Geometry: see drawing. Coordinates: mm, zero at the bounding-box minimum. A direction names the side the tool comes from. Give positions to 0.01 mm unless a question says otherwise; leave off trailing zeros. Write each loop counter-clockwise with the first axis right and the second up, starting at its lowest first coordinate (ties: lowest second). Pieces come first, ordered by that corner, then holes. Notation, with made-up numbers: (61.25, 33) -> (104.25, 33) arc R17 cw to (104.25, 54) -> close; hole circle Ø11 at (-9.75, -10.5). An arc over 180 degrees is marked (long way). Answer as a JSON object with one key per item and string values. Group by question number.
Item 1: Section query A-A on x = 4.5. Return the cut outline in (y, z).
Item 2: Section query C-C on y = 80. Return the cut outline in (x, z), plus the area to 3 significant figures.
Item 3: Access query for the marked faces 1 and 2. Directions: +Z, -Z, +X, -X, +Y, -Y. A direction counts if a zero-diameter tool reaches every point of the face in a straight line with its end or side. Return the directions, or none.
Item 4: First-contact query: pin 1 Ø10 at (x, y) = (35, 77.5) entering from +Z; pin 2 Ø5 at (x, y) = (39, 31.5) entering from +Z; pin 3 Ø20.5 at (x, z) = (37.5, 94) entering from -Y. Flat tips, straight axial feed; report the tip coordinate or a pass-through.
Item 5: Ray query, probe 1 along Y at (x, z) = (42, 86); probe 2 along Z at (x, y) = (31.5, 36); probe 3 along Y at (x, z) = (3, 72.5). Return the intervals inside material, ascending. Write a range as from..to.
Item 6: Section query B-B on z = 93.5. Return the cut outline in (x, y).
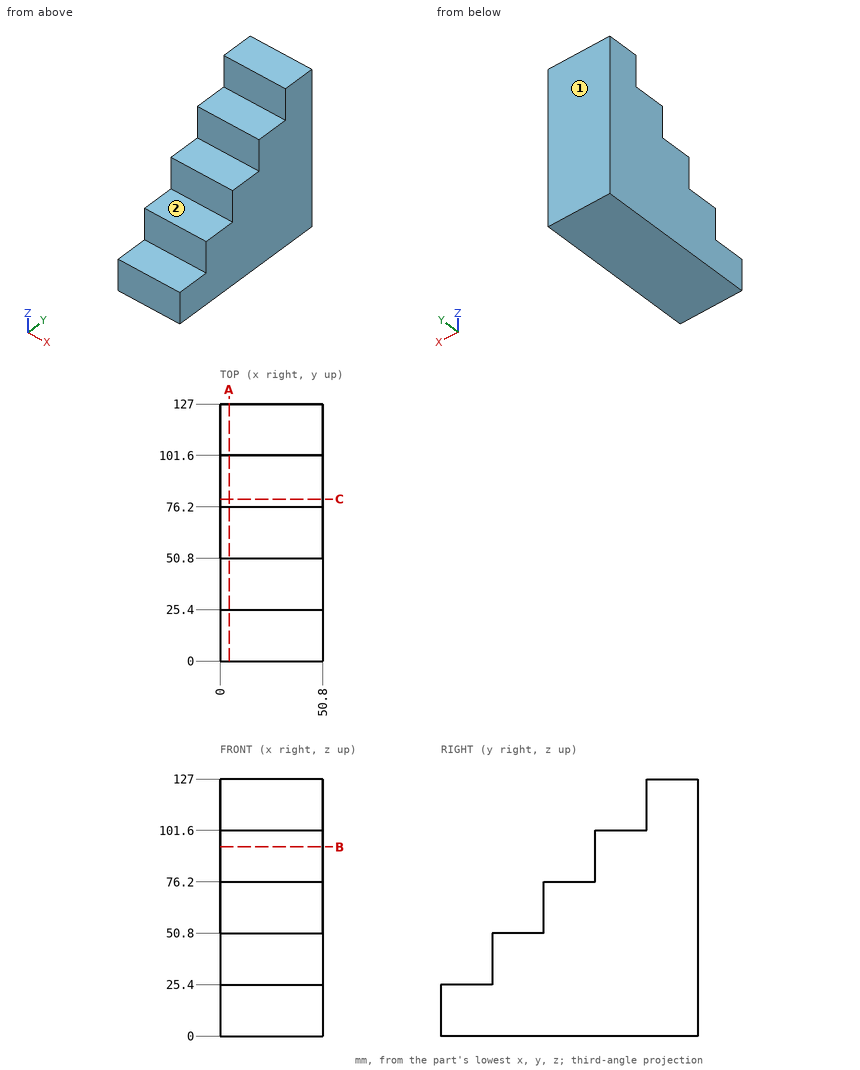
Worked answers:
{
 "1": {"outline": "(0, 0) -> (127, 0) -> (127, 127) -> (101.6, 127) -> (101.6, 101.6) -> (76.2, 101.6) -> (76.2, 76.2) -> (50.8, 76.2) -> (50.8, 50.8) -> (25.4, 50.8) -> (25.4, 25.4) -> (0, 25.4) -> close"},
 "2": {"outline": "(0, 0) -> (50.8, 0) -> (50.8, 101.6) -> (0, 101.6) -> close", "area": "5,160 mm^2"},
 "3": {"face 1": "+Z, -Z, +X, -X, +Y", "face 2": "+Z, +X, -X, -Y"},
 "4": {"pin 1": "z = 101.6", "pin 2": "z = 50.8", "pin 3": "y = 76.2"},
 "5": {"probe 1": "76.2..127", "probe 2": "0..50.8", "probe 3": "50.8..127"},
 "6": {"outline": "(0, 76.2) -> (50.8, 76.2) -> (50.8, 127) -> (0, 127) -> close"}
}
